Read the model definition and answer for the solid it produces. Units are mm, in the model's axes. A direction names the side the tool comes from. Coordinates: 2 decimals unless noted, no trailing zeros. Loops run counter-clockwise (first coordinate to the right, second up) from the corner with the lowest first, then second, coordinate; pieces in that order, holes last. Notation, with made-up numbers: (-0.5, 74.25) -> (31.5, 74.25) arc R12 cw to (31.5, 81.25) -> close; hole circle Ø7 at (83, -31). An arc over 180 degrees is marked (long way). Answer in a Markdown table with one row per item.
```python
from build123d import *

# Parameters (mm, degrees)
SKETCH_1_W          = 20.3
SKETCH_1_H          = 30.33
EXTRUDE_1_DEPTH     = 10
CUT_EXTRUDE_1_DEPTH = 28.240910869
SKETCH_3_R          = 1.6
CUT_EXTRUDE_2_DEPTH = 21.825740083
SKETCH_4_R          = 3.1
CUT_EXTRUDE_3_DEPTH = 8
SKETCH_5_R          = 0.95
CUT_EXTRUDE_4_DEPTH = 5
SKETCH_6_R          = 3.15
CUT_EXTRUDE_5_DEPTH = 3
FILLET_2_R          = 5


with BuildPart() as part:
    # 草图1 → 凸台-拉伸1 (new body)
    with BuildSketch(Plane(origin=(0, 0, 0), x_dir=(1, 0, 0), z_dir=(0, 1, 0))):
        with Locations((-0.035, 0)):
            Rectangle(SKETCH_1_W, SKETCH_1_H)
    extrude(amount=EXTRUDE_1_DEPTH)

    # 草图2 → 切除-拉伸1 (cut, through all)
    with BuildSketch(Plane.ZY.offset(10.185)):
        Polygon((-15.165, 6), (-9.85, 6), (-12.647845949, 0), (-15.165, 0), align=None)
        Polygon((12.647845949, 0), (9.85, 6), (15.165, 6), (15.165, 0), align=None)
    extrude(amount=-CUT_EXTRUDE_1_DEPTH, mode=Mode.SUBTRACT)

    # 草图3 → 切除-拉伸2 (cut, through all)
    with BuildSketch(Plane.XZ):
        with Locations(Location((0, 7, 0), (0, 0, 270))):
            Circle(SKETCH_3_R)
        with Locations(Location((7, 0, 0), (0, 0, 270))):
            Circle(SKETCH_3_R)
        with Locations(Location((0, -7, 0), (0, 0, 270))):
            Circle(SKETCH_3_R)
        with Locations(Location((-7, 0, 0), (0, 0, 270))):
            Circle(SKETCH_3_R)
    extrude(amount=-CUT_EXTRUDE_2_DEPTH, mode=Mode.SUBTRACT)

    # 草图4 → 切除-拉伸3 (cut)
    with BuildSketch(Plane.XZ):
        with Locations(Location((0, 7, 0), (0, 0, 270))):
            Circle(SKETCH_4_R)
        with Locations(Location((7, 0, 0), (0, 0, 270))):
            Circle(SKETCH_4_R)
        with Locations(Location((0, -7, 0), (0, 0, 270))):
            Circle(SKETCH_4_R)
        with Locations(Location((-7, 0, 0), (0, 0, 270))):
            Circle(SKETCH_4_R)
    extrude(amount=-CUT_EXTRUDE_3_DEPTH, mode=Mode.SUBTRACT)

    # 草图5 → 切除-拉伸4 (cut)
    with BuildSketch(Plane(origin=(10.115, 0, 0), x_dir=(0, 0, -1), z_dir=(1, 0, 0))):
        with Locations((-7.5, 3)):
            Circle(SKETCH_5_R)
        with Locations((7.5, 3)):
            Circle(SKETCH_5_R)
    extrude(amount=-CUT_EXTRUDE_4_DEPTH, mode=Mode.SUBTRACT)

    # 草图6 → 切除-拉伸5 (cut)
    with BuildSketch(Plane(origin=(0, 10, 0), x_dir=(1, 0, 0), z_dir=(0, 1, 0))):
        with Locations(Location((0, 0, 0), (0, 0, 270))):
            Circle(SKETCH_6_R)
    extrude(amount=-CUT_EXTRUDE_5_DEPTH, mode=Mode.SUBTRACT)

    # 圆角2
    fillet_2_edges = [part.edges().sort_by_distance(p)[0] for p in [
        (-10.185, 8, -15.165),
        (10.115, 8, -15.165),
        (10.115, 8, 15.165),
        (-10.185, 8, 15.165),
    ]]
    fillet(fillet_2_edges, radius=FILLET_2_R)


solid = part.part
```
1. A cutting plane is placed at C-C on y = 6.5. Give the vertices of the cut face in (x, z) (3 decimals).
A:
| item | result |
|---|---|
| outline | (-10.185, -10.165) arc R5 ccw to (-5.185, -15.165) -> (5.115, -15.165) arc R5 ccw to (10.115, -10.165) -> (10.115, 10.165) arc R5 ccw to (5.115, 15.165) -> (-5.185, 15.165) arc R5 ccw to (-10.185, 10.165) -> close; hole circle Ø6.2 at (-7, 0); hole circle Ø6.2 at (0, -7); hole circle Ø6.2 at (0, 7); hole circle Ø6.2 at (7, 0) |
2. Given pin 1 Ø1 at (y, z) = (6, -11.5) entering from -X; pin 2 Ø1.1 at (y, z) = (3, -7.5) entering from +X (3 decimals); pin 3 Ø3 at (x, z) = (-0.5, 0.5) entering from +Y, each flat-ended and moving along its own axis, determine where each tip first touches the part or whether it passes through.
A:
| item | result |
|---|---|
| pin 1 | stops at x = -10.11 |
| pin 2 | stops at x = 5.115 |
| pin 3 | stops at y = 7 |
3. A cutting plane is placed at A-A on z = 0. Give the vertices of the cut face in (x, y) (3 decimals), and give its area (3 significant figures).
A:
| item | result |
|---|---|
| outline | (-10.185, 0) -> (-10.1, 0) -> (-10.1, 8) -> (-8.6, 8) -> (-8.6, 10) -> (-10.185, 10) -> close; (-5.4, 8) -> (-3.9, 8) -> (-3.9, 0) -> (3.9, 0) -> (3.9, 8) -> (5.4, 8) -> (5.4, 10) -> (3.15, 10) -> (3.15, 7) -> (-3.15, 7) -> (-3.15, 10) -> (-5.4, 10) -> close; (8.6, 8) -> (10.1, 8) -> (10.1, 0) -> (10.115, 0) -> (10.115, 10) -> (8.6, 10) -> close |
| area | 72.1 mm2 |
4. The mould has two halves that part along Y. Classify faces 1 (the flat face through (-1.3, 8, -8.3)), 2 (the cylindrical face through (7.65, 3.04, -6.55)), 3 (the cylindrical face through (-8.76, 8.03, -13.66)): pulls with the +Y half, pulls with the -Y half, needs draft (parallel to the pull), parting line crosses it, or undercut.
A:
| item | result |
|---|---|
| face 1 | pulls with the -Y half |
| face 2 | undercut |
| face 3 | needs draft |
5. A cutting plane is placed at B-B on x = 7. Give the vertices of the cut face in (y, z).
A:
| item | result |
|---|---|
| outline | (0, -12.65) -> (6, -9.85) -> (6, -14.8) -> (10, -14.8) -> (10, -1.6) -> (8, -1.6) -> (8, -3.1) -> (0, -3.1) -> close; (0, 3.1) -> (8, 3.1) -> (8, 1.6) -> (10, 1.6) -> (10, 14.8) -> (6, 14.8) -> (6, 9.85) -> (0, 12.65) -> close; hole circle Ø1.9 at (3, -7.5); hole circle Ø1.9 at (3, 7.5) |
6. A cutting plane is placed at D-D on x = 0. Count the separate pieces of the cut face and the enclosed holes in it, and give its area (3 significant figures).
A:
| item | result |
|---|---|
| separate pieces | 5 |
| enclosed holes | 0 |
| area | 126 mm2 |
7. A tool of negligible diameter and unlimited length cuts with its end or side. For faces 4 (the cylindrical face through (-8.76, 8.03, 13.66)), 5 (the flat face through (-8.3, 8, -1.3)), 6 (the cylindrical face through (-1.917, 8.521, -2.5)), from which of +Z, -Z, +X, -X, +Y, -Y can it reach the whole face along a straight path? Write none if from no direction.
A:
| item | result |
|---|---|
| face 4 | +Z, -X, +Y |
| face 5 | -Y |
| face 6 | +Y |
8. Find the intervals of material crossed by probe 1 along Y at (x, z) = (7.55, 7.5); probe 2 along X at (y, z) = (4.75, 7) (3 decimals); probe 3 along X at (y, z) = (5.25, 1) (3 decimals), in increasing order.
A:
| item | result |
|---|---|
| probe 1 | y = 0 to 2.05, 3.95 to 10 |
| probe 2 | x = -10.185 to -3.1, 3.1 to 10.115 |
| probe 3 | x = -10.185 to -9.934, -4.066 to 4.066, 9.934 to 10.115 |
